from build123d import *

# Parameters (mm, degrees)
SKETCH1_W           = 12
SKETCH1_H           = 6
BOSS_EXTRUDE1_DEPTH = 0.25
CUT_EXTRUDE1_DEPTH  = 0.125
SKETCH2_W           = 0.3
SKETCH2_H           = 0.25
BOSS_EXTRUDE2_DEPTH = 1
SKETCH4_W           = 4.136186254
SKETCH4_H           = 2.43263025
BOSS_EXTRUDE3_DEPTH = 0.25
FILLET2_R           = 0.1
CHAMFER1_SIZE       = 0.1
FILLET3_R           = 0.125
CHAMFER2_SIZE       = 0.1
FILLET4_R           = 0.125


with BuildPart() as part:
    # Sketch1 → Boss-Extrude1 (new body)
    with BuildSketch(Plane(origin=(0, 0, 0), x_dir=(1, 0, 0), z_dir=(0, 1, 0))):
        Rectangle(SKETCH1_W, SKETCH1_H)
    extrude(amount=BOSS_EXTRUDE1_DEPTH)

    # 3DSketch1 → Cut-Extrude1 (cut)
    with BuildSketch(Plane(origin=(-5.875, 0.25, -2.875), x_dir=(0.8982167220477767, 0, 0.43955286398082694), z_dir=(0, -1, 0))):
        Polygon((0, 0), (2.527428968, 5.164746152), (13.081475452, 0), (10.554046484, -5.164746152), align=None)
    extrude(amount=CUT_EXTRUDE1_DEPTH, mode=Mode.SUBTRACT)

    # Sketch2 → Boss-Extrude2 (add)
    with BuildSketch(Plane.XY.offset(3)):
        with Locations((-0.001421044, 0.125)):
            Rectangle(SKETCH2_W, SKETCH2_H)
    extrude(amount=BOSS_EXTRUDE2_DEPTH)

    # Sketch4 → Boss-Extrude3 (add)
    with BuildSketch(Plane.XY.offset(4)):
        with Locations((0, 0.125)):
            Rectangle(SKETCH4_W, SKETCH4_H)
    extrude(amount=BOSS_EXTRUDE3_DEPTH)

    # Fillet2
    fillet2_edges = [part.edges().sort_by_distance(p)[0] for p in [
        (2.068093127, 0.125, 4),
        (0, 1.341315125, 4),
        (-2.068093127, 0.125, 4),
        (0, -1.091315125, 4),
    ]]
    fillet(fillet2_edges, radius=FILLET2_R)

    # Chamfer1
    chamfer1_edges = [part.edges().sort_by_distance(p)[0] for p in [
        (2.068093127, 0.125, 4.25),
        (0, 1.341315125, 4.25),
        (-2.068093127, 0.125, 4.25),
        (0, -1.091315125, 4.25),
    ]]
    chamfer(chamfer1_edges, length=CHAMFER1_SIZE)

    # Fillet3
    fillet3_edges = [part.edges().sort_by_distance(p)[0] for p in [
        (0, 0.25, 2.875),
        (-5.875, 0.25, 0),
        (0, 0.25, -2.875),
        (5.875, 0.25, 0),
    ]]
    fillet(fillet3_edges, radius=FILLET3_R - 0.0001)  # a hair under: the kernel refuses the full size

    # Chamfer2
    chamfer2_edges = [part.edges().sort_by_distance(p)[0] for p in [
        (0.148578956, 0, 3.5),
        (0.148578956, 0.25, 3.5),
        (-0.151421044, 0.25, 3.5),
        (-0.151421044, 0, 3.5),
    ]]
    chamfer(chamfer2_edges, length=CHAMFER2_SIZE)

    # Fillet4
    fillet4_edges = [part.edges().sort_by_distance(p)[0] for p in [
        (6, 0, 0),
        (3.024289478, 0, 3),
        (-3.025710522, 0, 3),
        (-6, 0, 0),
        (0, 0, -3),
    ]]
    fillet(fillet4_edges, radius=FILLET4_R)


solid = part.part
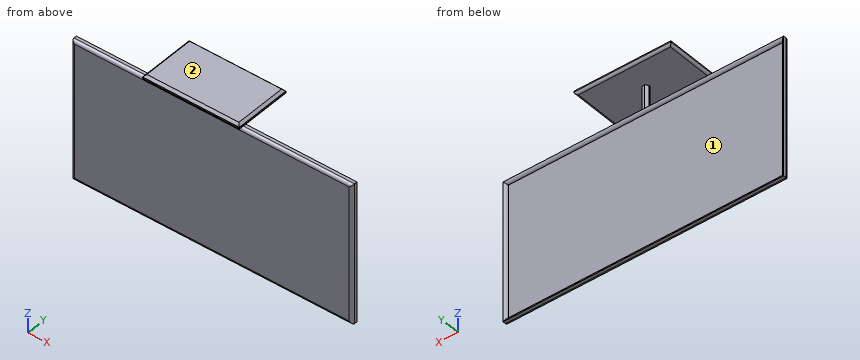
The listing builds one solid part. Answer for the finished solid, in the listing's coordinates (mm). Face numbers are marked on the shaded views. Round coordinates to 2 decimals unless told otherwise and drop trailing zeros. Loops run counter-clockwise (first coordinate to the right, second up) from the corner with the lowest first, then second, coordinate; pieces in that order, holes last. Notation, with made-up numbers: M -12,6.5 L 39,6.5 A28 cw 39,29.5 Z; hole C -10.5,-22 d2. An arc over 180 degrees is marked long. Return JSON: item names as keys, results as strings.
Q1. This flat-tipped pin is pushed along its axis until it touches: pin 1 Ø3 at (x, z) = (3.5, 0) entering from +Y (3 decimals). Where does it stop, or does it pass through?
Results list:
{"pin 1": "stops at y = 0.125"}
Q2. Find the intervals of material crossed by line 1 along Z through (x, y) = (-0.5, 0.95), in increasing order. Write a range as from..to.
Results list:
{"line 1": "z = 4..4.25"}
Q3. The mould has two halves that part along X. Classify the marked faces 1 and 2: released by +X, released by -X, zero draft, split by the parting line, or undercut.
Results list:
{"face 1": "undercut", "face 2": "zero draft"}
Q4. Find section D-D, the plane y = -0.4. Determine the outline of the cut face in (x, z).
Results list:
{"outline": "M -2.07,4.1 A0.1 ccw -1.97,4 L 1.97,4 A0.1 ccw 2.07,4.1 L 2.07,4.15 L 1.97,4.25 L -1.97,4.25 L -2.07,4.15 Z"}
